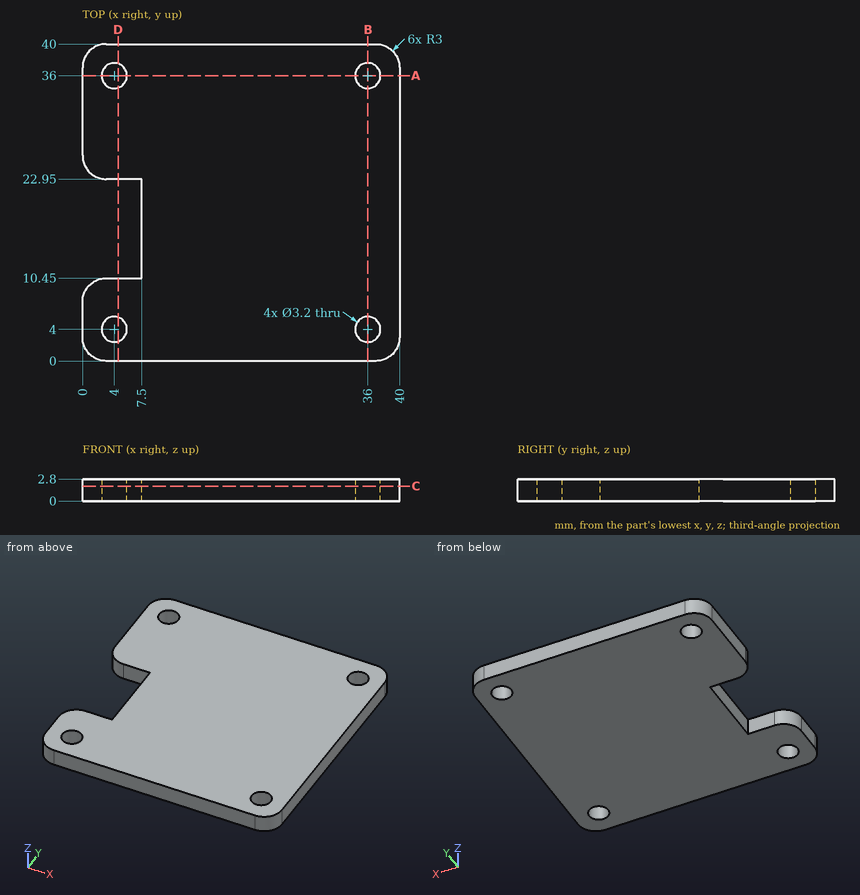
Print and shaded views of the part. All mm, measured from the part's lowest x, y and z. Coordinates: 2 decimals unless noted, no trailing zeros. Loops run counter-clockwise (first coordinate to the right, second up) from the corner with the lowest first, then second, coordinate; pieces in that order, holes last. Notation, with made-up numbers: (-37, 85) - (-30, 85) arc R12 ccw to (-30, 99) - close; hole circle Ø4 at (44.25, 14.25). An arc over 180 degrees is marked (long way). Use one line per item in the form item = value. Start each with the question number.
1) Band-saw the part on A-A (y = 36). Give the cut face in (x, z), and give its area (3 significant figures).
2) Band-saw the part on D-D (x = 4.5). Give the cut face in (y, z), and give its area (3 significant figures).
3) Flat gauge pins, fed straight in: pin 1 (1.9 mm diameter, centred on x = 36, y = 4, fed in from -Z); pin 2 (1 mm diameter, centred on y = 14.5, z = 1.5, fed in from -X); pin 3 (4 mm diameter, centred on x = 36, y = 36, fed in from -Z). Where does each tip first touch, or does it go through?
4) Band-saw the part on C-C (z = 1.9). Give the cut face in (x, y), and give its area (3 significant figures).
5) Drill centre lines: L1, parallel to Y at x = 36, z = 1.7; L2, parallel to Y at x = 4, z = 1.45; L3, parallel to Y at x = 36.5, z = 0.8. Where is each one in solid material? Low to high. Write a range as from..to.
Check values:
q1.outline = (0, 0) - (2.4, 0) - (2.4, 2.8) - (0, 2.8) - close; (5.6, 0) - (34.4, 0) - (34.4, 2.8) - (5.6, 2.8) - close; (37.6, 0) - (40, 0) - (40, 2.8) - (37.6, 2.8) - close
q1.area = 94.1 mm2
q2.outline = (0, 0) - (2.48, 0) - (2.48, 2.8) - (0, 2.8) - close; (5.52, 0) - (10.45, 0) - (10.45, 2.8) - (5.52, 2.8) - close; (22.95, 0) - (34.48, 0) - (34.48, 2.8) - (22.95, 2.8) - close; (37.52, 0) - (40, 0) - (40, 2.8) - (37.52, 2.8) - close
q2.area = 60.0 mm2
q3.pin_1 = through
q3.pin_2 = 7.5
q3.pin_3 = 0
q4.outline = (0, 3) arc R3 ccw to (3, 0) - (37, 0) arc R3 ccw to (40, 3) - (40, 37) arc R3 ccw to (37, 40) - (3, 40) arc R3 ccw to (0, 37) - (0, 25.95) arc R3 ccw to (3, 22.95) - (7.5, 22.95) - (7.5, 10.45) - (3, 10.45) arc R3 ccw to (0, 7.45) - close; hole circle Ø3.2 at (4, 4); hole circle Ø3.2 at (4, 36); hole circle Ø3.2 at (36, 4); hole circle Ø3.2 at (36, 36)
q4.area = 1,460 mm2
q5.L1 = 0..2.4, 5.6..34.4, 37.6..40
q5.L2 = 0..2.4, 5.6..10.45, 22.95..34.4, 37.6..40
q5.L3 = 0..2.48, 5.52..34.48, 37.52..40
